```python
from build123d import *

# Parameters (mm, degrees)
SKETCH_1_W               = 10
SKETCH_1_H               = 10
EXTRUDE_1_DEPTH          = 6
SKETCH_2_R               = 1.65
CUT_EXTRUDE_1_DEPTH      = 6
SKETCH_3_R               = 1.65
CUT_EXTRUDE_2_DEPTH      = 1
CUT_EXTRUDE_2_DEPTH_BACK = 11
SKETCH_4_R               = 1.65
CUT_EXTRUDE_3_DEPTH      = 11


with BuildPart() as part:
    # 草图1 → 凸台-拉伸1 (new body)
    with BuildSketch(Plane.XY):
        Rectangle(SKETCH_1_W, SKETCH_1_H)
    extrude(amount=EXTRUDE_1_DEPTH)

    # 草图2 → 切除-拉伸1 (cut)
    with BuildSketch(Plane.XY.offset(6)):
        Circle(SKETCH_2_R)
    extrude(amount=-CUT_EXTRUDE_1_DEPTH, mode=Mode.SUBTRACT)

    # 草图3 → 切除-拉伸2 (cut, two sides)
    with BuildSketch(Plane.ZY.offset(5)) as cut_extrude_2_sk:
        with Locations((3, 0)):
            Circle(SKETCH_3_R)
    extrude(amount=CUT_EXTRUDE_2_DEPTH, mode=Mode.SUBTRACT)
    extrude(cut_extrude_2_sk.sketch, amount=-CUT_EXTRUDE_2_DEPTH_BACK, mode=Mode.SUBTRACT)

    # 草图4 → 切除-拉伸3 (cut, through all)
    with BuildSketch(Plane(origin=(0, 5, 0), x_dir=(1, 0, 0), z_dir=(0, 1, 0))):
        with Locations((0, -3)):
            Circle(SKETCH_4_R)
    extrude(amount=-CUT_EXTRUDE_3_DEPTH, mode=Mode.SUBTRACT)


solid = part.part
```
Check sheet for the modelled part. Datum: model origin and axes. Units: mm. Give positions to 0.01 mm unless a question says otherwise; leave off trailing zeros. Order: outer loops, then holes, each group sorted by start corner. A loop starts at its lowest first (then second) coordinate and runs counter-clockwise, first axis right, second up. Notation, with made-up numbers: M 88.25,0.25 L 121.25,0.25 A29 ccw 121.25,29.25 Z; hole C 52,-0.5 d5. An arc over 180 degrees is marked long. Answer in a Markdown table with one row per item. Add a question column.
Q1. Thickness scan on L1, parallel to Z at x = 0, y = -2.75; L2, parallel to Y at x = 0, z = 0.3; L3, parallel to Y at x = 1.5, z = 1.05. Record the ranges inside material, lowest first.
Q2. Release check for a two-part mould opening along Z. For faces 1 (the flat face through (5, -1.2, 1.6)), 2 (the flat face through (0, 2, 6)), 3 (the flat face through (0, 2, 0)), 4 (the cylindrical face through (-1.216, 3.11, 1.885)) record: released by +Z, released by -Z, zero draft, split by the parting line, or undercut.
Q3. Sectioned sample at C-C, the plane y = 2.25. Record the boundary of the cut face in (x, z).
Q4. Gauge pin test, flat end, axial feed: pin 1 Ø3 at (x, z) = (0, 3) entering from +Y. Record the tip position at first contact, or that the pin passes through.
Q5. Sectioned sample at A-A, the plane z = 3. Record the boundary of the cut face in (x, y).
Q6. Sectioned sample at B-B, the plane x = 0. Record the boundary of the cut face in (y, z), and give its area (3 significant figures).
Verdict:
| question | item | result |
|---|---|---|
| 1 | L1 | 0 to 1.35, 4.65 to 6 |
| 1 | L2 | -5 to -1.65, 1.65 to 5 |
| 1 | L3 | -5 to -0.69, 0.69 to 5 |
| 2 | face 1 | zero draft |
| 2 | face 2 | released by +Z |
| 2 | face 3 | released by -Z |
| 2 | face 4 | undercut |
| 3 | outline | M -5,0 L 5,0 L 5,6 L -5,6 Z; hole C 0,3 d3.3 |
| 4 | pin 1 | through |
| 5 | outline | M -5,-5 L -1.65,-5 L -1.65,-1.65 L -5,-1.65 Z; M -5,1.65 L -1.65,1.65 L -1.65,5 L -5,5 Z; M 1.65,-5 L 5,-5 L 5,-1.65 L 1.65,-1.65 Z; M 1.65,1.65 L 5,1.65 L 5,5 L 1.65,5 Z |
| 6 | outline | M -5,0 L -1.65,0 L -1.65,1.35 L -5,1.35 Z; M -5,4.65 L -1.65,4.65 L -1.65,6 L -5,6 Z; M 1.65,0 L 5,0 L 5,1.35 L 1.65,1.35 Z; M 1.65,4.65 L 5,4.65 L 5,6 L 1.65,6 Z |
| 6 | area | 18.1 mm² |
